Could you check a few things on this model? Use its own coordinates, in mm. A direction names the side the tool comes from. Give positions to 0.01 mm unless a question says otherwise; leave off trailing zeros. Loops run counter-clockwise (first coordinate to the right, second up) from the corner with the lowest first, then second, coordinate; pieces in that order, holes last. Notation, with made-up numbers: M 39.5,-18.5 L 61.5,-18.5 A21 cw 61.5,15.5 Z; hole C 85,19.5 d6. An arc over 180 degrees is marked long. Write each question's results on one line, items separated by ' | '. Start each with the question number.
from build123d import *

# Parameters (mm, degrees)
SKETCH1_W                                    = 100
SKETCH1_H                                    = 68
BOSS_EXTRUDE1_DEPTH                          = 12.5
CBORE_FOR_M6_HEX_HEAD_CAP_SCREW1_D           = 6.6
CBORE_FOR_M6_HEX_HEAD_CAP_SCREW1_CBORE_D     = 14.547
CBORE_FOR_M6_HEX_HEAD_CAP_SCREW1_CBORE_DEPTH = 6
FILLET1_R                                    = 8
FILLET2_R                                    = 2


with BuildPart() as part:
    # Sketch1 → Boss-Extrude1 (new body)
    with BuildSketch(Plane(origin=(0, 0, 0), x_dir=(1, 0, 0), z_dir=(0, 1, 0))):
        with Locations((50, -34)):
            Rectangle(SKETCH1_W, SKETCH1_H)
    extrude(amount=BOSS_EXTRUDE1_DEPTH)

    # CBORE for M6 Hex Head Cap Screw1 (through all)
    with Locations(Plane(origin=(36.15, 0, 49), x_dir=(0, 0, -1), z_dir=(0, -1, 0))):
        with Locations((0, 0), (30, 0), (0, 27.7), (30, 27.7)):
            CounterBoreHole(CBORE_FOR_M6_HEX_HEAD_CAP_SCREW1_D / 2, CBORE_FOR_M6_HEX_HEAD_CAP_SCREW1_CBORE_D / 2, CBORE_FOR_M6_HEX_HEAD_CAP_SCREW1_CBORE_DEPTH)

    # Fillet1
    fillet1_edges = [part.edges().sort_by_distance(p)[0] for p in [
        (100, 12.5, 34),
        (50, 12.5, 0),
        (0, 12.5, 34),
        (50, 12.5, 68),
        (0, 6.25, 0),
        (100, 6.25, 0),
        (100, 6.25, 68),
        (0, 6.25, 68),
    ]]
    fillet(fillet1_edges, radius=FILLET1_R)

    # Fillet2
    fillet2_edges = [part.edges().sort_by_distance(p)[0] for p in [
        (100, 0, 34),
        (0, 0, 34),
        (50, 0, 0),
        (50, 0, 68),
        (97.656854249, 0, 2.343145751),
        (2.343145751, 0, 65.656854249),
        (2.343145751, 0, 2.343145751),
        (97.656854249, 0, 65.656854249),
    ]]
    fillet(fillet2_edges, radius=FILLET2_R)


solid = part.part
1) Thinking about a two-plate mould opening in X: for faces 3 (the face through (99.4, 0.57, 33.64)), 4 (the face through (49, 3, 68)), 5 (the face through (57.4, 2.96, 45.64)), which applies, pulls with the +X half, pulls with the -X half, needs draft (parallel to the pull), parting line crosses it, or undercut?
2) Which directions (+Z, -Z, +X, -X, +Y, -Y) give clear straight access to the entire face, cutting with the end or side of a thin tool? Please do faces 1 (the face through (62, 6, 46)), 2 (the face through (34.142, 9.296, 46.381)).
3) If we section it at B-B on z = 19: Write out the boundary of the cut face in (x, y).
4) If we section it at C-C on z = 39: Write out the boundary of the cut face in (x, y), plus the area to 3 significant figures.
5) If we section it at D-D on x = 76.5: Write out the boundary of the cut face in (y, z), plus the area to 3 significant figures.
6) Please list where these lines run through material, in increasing order: line 1 (X direction, y = 2.25, z = 48.5); line 2 (X direction, y = 10.5, z = 49); line 3 (Z direction, x = 66, y = 2). Write a range as from..to.
7) If we section it at A-A on x = 36.15: Write out the boundary of the cut face in (y, z), plus the area to 3 significant figures.
8) I'm going to push flat-ended pins straight in: P1, Ø23.5, axis at x = 36.15, z = 19, coming from the -Y side; P2, Ø11.5, axis at x = 64.5, z = 48.5, coming from the -Y side. Where does each tip first touch, or does it pass through?
Calculated:
1) face 3: pulls with the +X half | face 4: needs draft | face 5: undercut
2) face 1: -Y | face 2: +Y, -Y
3) outline: M 0,2 A2 ccw 2,0 L 28.88,0 L 28.88,6 L 32.85,6 L 32.85,12.5 L 8,12.5 A8 ccw 0,4.5 Z; M 39.45,6 L 43.42,6 L 43.42,0 L 56.58,0 L 56.58,6 L 60.55,6 L 60.55,12.5 L 39.45,12.5 Z; M 67.15,6 L 71.12,6 L 71.12,0 L 98,0 A2 ccw 100,2 L 100,4.5 A8 ccw 92,12.5 L 67.15,12.5 Z
4) outline: M 0,2 A2 ccw 2,0 L 98,0 A2 ccw 100,2 L 100,4.5 A8 ccw 92,12.5 L 8,12.5 A8 ccw 0,4.5 Z | area: 1,220 mm2
5) outline: M 0,2 A2 ccw 2,0 L 4.5,0 A8 ccw 12.5,8 L 12.5,60 A8 ccw 4.5,68 L 2,68 A2 ccw 0,66 Z | area: 821 mm2
6) line 1: x = 0..28.89, 43.41..56.59, 71.11..100 | line 2: x = 2.71..32.85, 39.45..60.55, 67.15..97.29 | line 3: z = 0..12.05, 25.95..42.05, 55.95..68
7) outline: M 0,2 A2 ccw 2,0 L 4.5,0 A8 ccw 12.5,8 L 12.5,15.7 L 6,15.7 L 6,11.73 L 0,11.73 Z; M 0,26.27 L 6,26.27 L 6,22.3 L 12.5,22.3 L 12.5,45.7 L 6,45.7 L 6,41.73 L 0,41.73 Z; M 0,56.27 L 6,56.27 L 6,52.3 L 12.5,52.3 L 12.5,60 A8 ccw 4.5,68 L 2,68 A2 ccw 0,66 Z | area: 560 mm2
8) P1: stops at y = 0 | P2: stops at y = 6
